Design review of the part shown in the three views and the two pictorial views. Dimensions are in mm from the part's minimum x, y and z. Give positions to 0.01 mm unless a question says otherwise; leave off trailing zeros. Loops run counter-clockwise (first coordinate to the right, second up) from the corner with the lowest first, then second, coordinate; pieces in that order, holes last. Notation, with made-up numbers: (-27, 52.5) -> (13, 52.5) arc R32 cw to (13, 88.5) -> close; hole circle Ø5 at (54, -20.5). An arc over 180 degrees is marked (long way). Answer as CSV lines item,"result". Start each with the question number.
Item 1: Add section B-B on x = 31.5. State the section outline as (y, z) points.
Item 2: Add section D-D on y = 14.5. State the section outline as (x, z) points.
Item 3: Clearance check with flat-ended pins moving along their axes: P1, Ø1, axis at x = 6, y = 3, coming from the -Z side; P2, Ø12, axis at x = 16, z = 20.5, coming from the +Y side; P3, Ø2.5, axis at y = 2.33, z = 20, coming from the -X side; P4, Ø12, axis at y = 18, z = 5.5, coming from the +X side. State where each tip first meets the part, or that it passes through.
Item 4: Add section C-C on z = 34.75. State the section outline as (x, y) points, plus the area to 3 significant figures.
Item 5: For L1, parallel to Y at x = 40.95, z = 20; L2, parallel to X at y = 13.25, z = 12.5; L3, parallel to Y at x = 1, z = 20, list the stretches that pass through material, from the lowest coordinate up. Write a range as from..to.
Item 6: Add section A-A on z = 20. State the section outline as (x, y) points, plus the area to 3 significant figures.
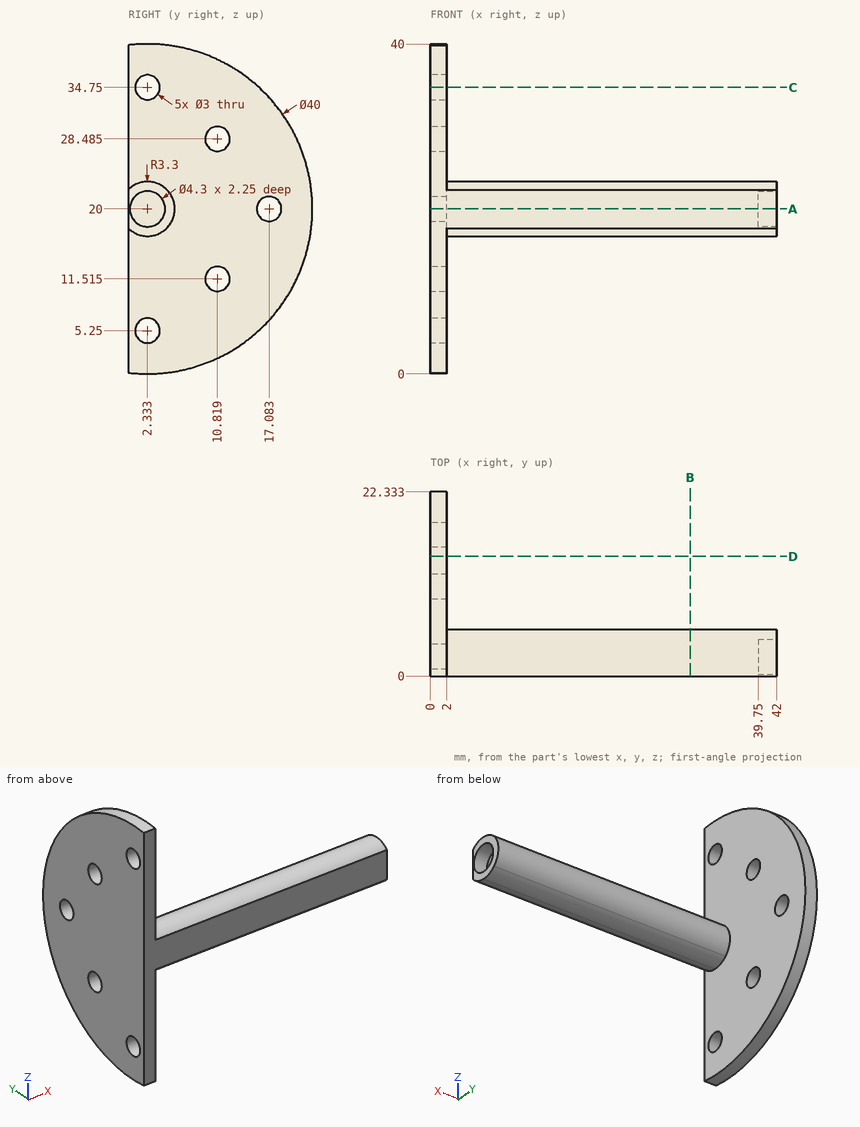
Computed values:
1,outline,"(0, 17.67) arc R3.3 ccw (long way) to (0, 22.33) -> close"
2,outline,"(0, 4.13) -> (2, 4.13) -> (2, 35.87) -> (0, 35.87) -> close"
3,P1,"z = 16.7"
3,P2,"y = 5.63"
3,P3,"x = 0"
3,P4,"x = 2"
4,outline,"(0, 0) -> (2, 0) -> (2, 0.83) -> (0, 0.83) -> close; (0, 3.83) -> (2, 3.83) -> (2, 15.84) -> (0, 15.84) -> close"
4,area,"25.7 mm²"
5,L1,"0..0.18, 4.48..5.63"
5,L2,"0..2"
5,L3,"0..15.58, 18.58..22.33"
6,outline,"(0, 0) -> (42, 0) -> (42, 0.18) -> (39.75, 0.18) -> (39.75, 4.48) -> (42, 4.48) -> (42, 5.63) -> (2, 5.63) -> (2, 15.58) -> (0, 15.58) -> close; (0, 18.58) -> (2, 18.58) -> (2, 22.33) -> (0, 22.33) -> close"
6,area,"254 mm²"
